```python
from build123d import *

# Parameters (mm, degrees)
SKETCH1_R           = 6.35
BOSS_EXTRUDE1_DEPTH = 7.9375
BOSS_EXTRUDE2_DEPTH = 104.6734
SKETCH3_R           = 6.35
BOSS_EXTRUDE3_DEPTH = 7.9375


with BuildPart() as part:
    # Sketch1 → Boss-Extrude1 (new body)
    with BuildSketch(Plane.XY):
        Circle(SKETCH1_R)
    extrude(amount=BOSS_EXTRUDE1_DEPTH)

    # Sketch2 → Boss-Extrude2 (add)
    with BuildSketch(Plane.XY.offset(7.9375)):
        Polygon((7.332348419, 0), (3.666174209, 6.35), (-3.666174209, 6.35), (-7.332348419, 0), (-3.666174209, -6.35), (3.666174209, -6.35), align=None)
    extrude(amount=BOSS_EXTRUDE2_DEPTH)

    # Sketch3 → Boss-Extrude3 (add)
    with BuildSketch(Plane.XY.offset(112.6109)):
        with Locations(Location((0, 0, 0), (0, 0, 150))):
            Circle(SKETCH3_R)
    extrude(amount=BOSS_EXTRUDE3_DEPTH)


solid = part.part
```
Can you work these out from the model? Positions are in its coordinate system, mm. A direction names the side the tool comes from. Give positions to 0.01 mm unless a question says otherwise; leave off trailing zeros. Loops run counter-clockwise (first coordinate to the right, second up) from the corner with the lowest first, then second, coordinate; pieces in that order, holes last. Notation, with made-up numbers: M 61.5,4.25 L 102.5,4.25 A30 ccw 102.5,35.25 Z; hole C -8.75,79 d9. An arc over 180 degrees is marked long. Use one line per item in the form item = value. Start each with the question number.
(1) I want a section at A-A, the plane z = 15. Write out the boundary of the cut face in (x, y), and give its area (3 significant figures).
(2) Please list where these lines run through material, in increasing order: line 1 (Y direction, x = -5.5, z = 56.5); line 2 (X direction, y = -0.25, z = 89.5); line 3 (X direction, y = -3.5, z = 68).
(3) I want a section at B-B, the plane y = 4.5. Write out the boundary of the cut face in (x, z).
(4) I want a section at C-C, the plane y = -4.75. Write out the boundary of the cut face in (x, z), and give its area (3 significant figures).
(5) On a 3-axis mill with a long thin cutter (end or side, diameter ignored), from which of +Z, -Z, +X, -X, +Y, -Y can I reach the whole of each face in a straight line? I mean faces 1 (the flat face through (3, 6, 7.938)), 2 (the flat face through (-3, -6, 112.611)), 3 (the cylindrical face through (-1.38, -6.2, 3.91)), 4 (the flat face through (7, 0, 7.938)). Say none if no direction works.
(6) I'm going to push flat-ended pins straight in: P1, Ø4, axis at y = 3.5, z = 103, coming from the -X side; P2, Ø1, axis at y = 1.5, z = 74.5, coming from the +X side (3 decimals). Where does each tip first touch, or does it pass through?
Worked out:
q1.outline = M -7.33,0 L -3.67,-6.35 L 3.67,-6.35 L 7.33,0 L 3.67,6.35 L -3.67,6.35 Z
q1.area = 140 mm²
q2.line_1 = -3.17 to 3.17
q2.line_2 = -7.19 to 7.19
q2.line_3 = -5.31 to 5.31
q3.outline = M -4.73,7.94 L -4.48,7.94 L -4.48,0 L 4.48,0 L 4.48,7.94 L 4.73,7.94 L 4.73,112.61 L 4.48,112.61 L 4.48,120.55 L -4.48,120.55 L -4.48,112.61 L -4.73,112.61 Z
q4.outline = M -4.59,7.94 L -4.21,7.94 L -4.21,0 L 4.21,0 L 4.21,7.94 L 4.59,7.94 L 4.59,112.61 L 4.21,112.61 L 4.21,120.55 L -4.21,120.55 L -4.21,112.61 L -4.59,112.61 Z
q4.area = 1,090 mm²
q5.face_1 = -Z, +X, +Y
q5.face_2 = +Z, -X, -Y
q5.face_3 = -Z
q5.face_4 = -Z, +X
q6.P1 = -6.47
q6.P2 = 6.755
